The figure shows three views and two pictorial views of one solid part (mm, origin at its lowest corner). Answer the questions. Round coordinates to 2 decimals unless told otherwise and drop trailing zeros. Order: outer loops, then holes, each group sorted by start corner. A loop starts at its lowest first (then second) coordinate and runs counter-clockwise, first axis right, second up. Notation, with made-up numbers: (49, 5.5) - (106, 5.5) arc R13 ccw to (106, 30.5) - close; hole circle Ø11 at (80, 32.25). An arc over 180 degrees is marked (long way). Answer as a JSON object with one key per item and string values. Group by question number.
Q1. Consider line 1 (X direction, y = 0.8, z = 2.5); line 2 (Z direction, x = 29, y = 0.2); line 3 (X direction, y = 1.25, z = 3.5). Determine where each line is inside the solid, lowest interval first.
Q2. A cutting plane is placed at A-A on z = 2.5. Determine the outline of the cut face in (x, y).
Q3. A cutting plane is placed at B-B on x = 2.5. Determine the outline of the cut face in (y, z).
Q4. A cutting plane is placed at C-C on y = 0.5. Determine the outline of the cut face in (x, z), and give its area (3 significant figures).
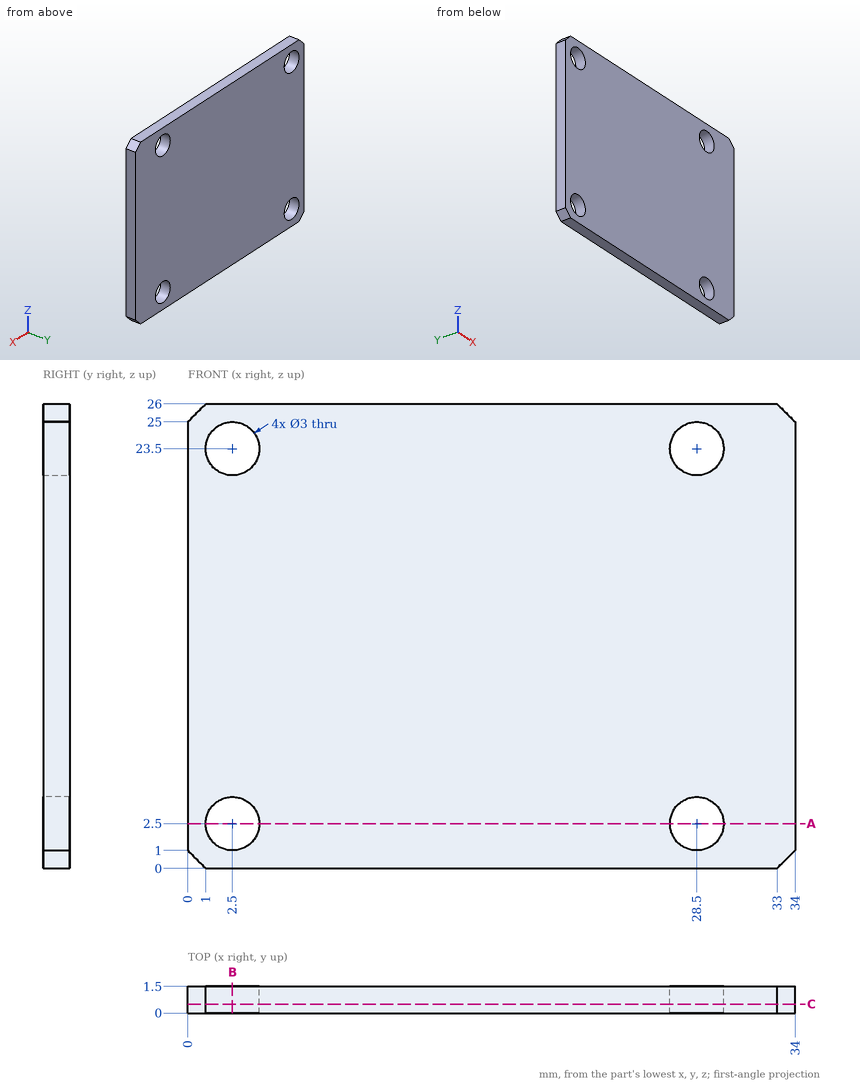
Result set:
{
 "1": {"line 1": "x = 0 to 1, 4 to 27, 30 to 34", "line 2": "z = 0 to 1.09, 3.91 to 22.09, 24.91 to 26", "line 3": "x = 0 to 1.38, 3.62 to 27.38, 29.62 to 34"},
 "2": {"outline": "(0, 0) - (1, 0) - (1, 1.5) - (0, 1.5) - close; (4, 0) - (27, 0) - (27, 1.5) - (4, 1.5) - close; (30, 0) - (34, 0) - (34, 1.5) - (30, 1.5) - close"},
 "3": {"outline": "(0, 0) - (1.5, 0) - (1.5, 1) - (0, 1) - close; (0, 4) - (1.5, 4) - (1.5, 22) - (0, 22) - close; (0, 25) - (1.5, 25) - (1.5, 26) - (0, 26) - close"},
 "4": {"outline": "(0, 1) - (1, 0) - (33, 0) - (34, 1) - (34, 25) - (33, 26) - (1, 26) - (0, 25) - close; hole circle Ø3 at (2.5, 2.5); hole circle Ø3 at (2.5, 23.5); hole circle Ø3 at (28.5, 2.5); hole circle Ø3 at (28.5, 23.5)", "area": "854 mm²"}
}
